Could you check a few things on this model? Use its own coordinates, in mm. Face numbers are marked on the shaded views. Round coordinates to 2 decimals unless told otherwise and drop trailing zeros. Loops run counter-clockwise (first coordinate to the right, second up) from the corner with the lowest first, then second, coordinate; pieces in that order, holes last. Notation, with made-up numbers: (78.25, 80.25) -> (110.25, 80.25) arc R6 cw to (110.25, 91.25) -> close; hole circle Ø6 at (-29.5, 32.5). An arc over 180 degrees is marked (long way). One line per item, written item: value.
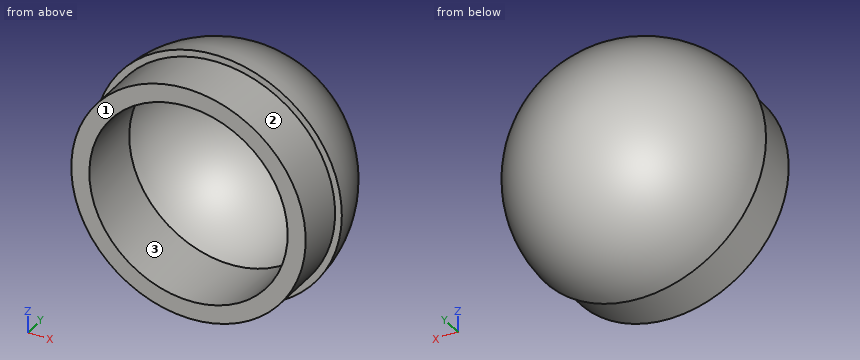
```python
from build123d import *

# Parameters (mm, degrees)
F2_T = -2


with BuildPart() as f1:
    # F0 (on Right) → F1 (revolve)
    with BuildSketch(Plane.YZ):
        with BuildLine():
            Line((5.5872295052, 12.9911601543), (0, 12.9911601543))
            Line((0, 12.9911601543), (0, 0))
            Line((0, 0), (18.7855159319, 0))
            ThreePointArc((18.7855159319, 0), (14.9512416834, 9.5247982797), (5.5872295052, 13.7365339324))
            Line((5.5872295052, 13.7365339324), (5.5872295052, 12.9911601543))
        make_face()
    revolve(axis=Axis((0, 9.392757966, 0), (0, -1, 0)))

    # F2
    f2_openings = [f1.faces().sort_by_distance(p)[0] for p in [
        (0, 0, 0),
    ]]
    offset(amount=F2_T, openings=f2_openings, kind=Kind.INTERSECTION)


solid = f1.part
```
Item 1: If we section it at A-A on x = 0: List the corners of the cut face in (y, z) for me, plus the area to 3 significant figures.
Output:
outline: (0, -12.99) -> (5.59, -12.99) -> (5.59, -13.74) arc R13.75 ccw to (5.59, 13.74) -> (5.59, 12.99) -> (0, 12.99) -> (0, 10.99) -> (7.59, 10.99) -> (7.59, 11.47) arc R11.75 cw to (7.59, -11.47) -> (7.59, -10.99) -> (0, -10.99) -> close
area: 103 mm²
Item 2: If we section it at D-D on y = 7: List the corners of the cut face in (x, z) for me.
Output:
outline: circle Ø27.21 at (0, 0); hole circle Ø21.98 at (0, 0)
Item 3: I need wall thicknesses on line 1 (Z direction, x = 0, y = 4); line 2 (Z direction, x = 0.5, y = 7.5). Which ranges of each line are inside material? Lowest first, please. Write a range as from..to.
Output:
line 1: z = -12.99..-10.99, 10.99..12.99
line 2: z = -13.52..-10.98, 10.98..13.52
Item 4: If we mould it in two halves opening along X, with no side actions, what happens to the marked faces 1, 2 and 3? For each: released by +X, released by -X, zero draft, split by the parting line, or undercut.
Output:
face 1: zero draft
face 2: split by the parting line
face 3: undercut
Item 5: Will these pins go through, and if not, where does the flat tip stop? pin 1 Ø7 at (x, z) = (5.5, 5.5) entering from +Y; pin 2 Ø4 at (x, z) = (5, 7) entering from +Y; pin 3 Ø2 at (x, y) = (-5.5, 3.5) entering from -Z.
Output:
pin 1: stops at y = 18.1
pin 2: stops at y = 17.1
pin 3: stops at z = -12.19
Item 6: If we section it at C-C on y = 3.75: List the corners of the cut face in (x, z) for me, plus the area to 3 significant figures.
Output:
outline: circle Ø25.98 at (0, 0); hole circle Ø21.98 at (0, 0)
area: 151 mm²
Item 7: If we section it at B-B on z = 0: List the corners of the cut face in (x, y) for me.
Output:
outline: (-13.74, 5.59) -> (-12.99, 5.59) -> (-12.99, 0) -> (-10.99, 0) -> (-10.99, 7.59) -> (-11.47, 7.59) arc R11.75 cw to (11.47, 7.59) -> (10.99, 7.59) -> (10.99, 0) -> (12.99, 0) -> (12.99, 5.59) -> (13.74, 5.59) arc R13.75 ccw to start
